from build123d import *

# Parameters (mm, degrees)
SKETCH1_W                    = 370
SKETCH1_H                    = 180
BOSS_EXTRUDE1_DEPTH          = 18
CONVERT_SOLID1_START         = -90
CONVERT_SOLID1_DEPTH         = 180
CONVERT_SOLID1_START_2       = -92
CONVERT_SOLID1_2_DEPTH       = 3.5
CONVERT_SOLID1_START_3       = 88.5
CONVERT_SOLID1_3_DEPTH       = 3.5
CONVERT_SOLID1_START_4       = -88.5
CONVERT_SOLID1_4_DEPTH       = 177
CONVERT_SOLID1_START_5       = -89
CONVERT_SOLID1_5_OUTLINE_W   = 367
CONVERT_SOLID1_5_OUTLINE_H   = 2
CONVERT_SOLID1_5_OUTLINE_W_2 = 2
CONVERT_SOLID1_5_OUTLINE_H_2 = 34.5
CONVERT_SOLID1_5_DEPTH       = 178
CONVERT_SOLID1_START_6       = -89.292893219
CONVERT_SOLID1_6_OUTLINE_W   = 2
CONVERT_SOLID1_6_OUTLINE_H   = 34.5
CONVERT_SOLID1_6_DEPTH       = 178.585786438
CONVERT_SOLID1_START_7       = -183.5
CONVERT_SOLID1_7_DEPTH       = 367
CONVERT_SOLID1_START_8       = -184.292893219
CONVERT_SOLID1_8_OUTLINE_W   = 2
CONVERT_SOLID1_8_OUTLINE_H   = 34.5
CONVERT_SOLID1_8_DEPTH       = 368.585786438
SKETCH6_W                    = 160
SKETCH6_H                    = 140
CUT_EXTRUDE1_DEPTH           = 36


with BuildPart() as part:
    # Sketch1 → Boss-Extrude1 (new, symmetric)
    with BuildSketch(Plane.XY):
        Rectangle(SKETCH1_W, SKETCH1_H)
    extrude(amount=BOSS_EXTRUDE1_DEPTH, both=True)

    # Convert-Solid1: read off the stored shape, not the designer's step
    # Convert-Solid1 outline → Convert-Solid1 (cut)
    with BuildSketch(Plane(origin=(0, 0, 0), x_dir=(1, 0, 0), z_dir=(0, 1, 0)).offset(CONVERT_SOLID1_START)):
        with BuildLine():
            ThreePointArc((-184, 18), (-184.707106781, 17.707106781), (-185, 17))
            Line((-185, 17), (-185, -18))
            Line((-185, -18), (185, -18))
            Line((185, -18), (185, 17))
            ThreePointArc((185, 17), (184.707106781, 17.707106781), (184, 18))
            Line((184, 18), (-184, 18))
        make_face()
    extrude(amount=CONVERT_SOLID1_DEPTH, mode=Mode.SUBTRACT)

    # Convert-Solid1 2 outline → Convert-Solid1 2 (cut)
    with BuildSketch(Plane(origin=(0, 0, 0), x_dir=(1, 0, 0), z_dir=(0, 1, 0)).offset(CONVERT_SOLID1_START_2)):
        with BuildLine():
            ThreePointArc((-185, 17), (-184.707106781, 17.707106781), (-184, 18))
            Line((-184, 18), (-185, 18))
            Line((-185, 18), (-185, 17))
        make_face()
        with BuildLine():
            Line((185, 18), (184, 18))
            ThreePointArc((184, 18), (184.707106781, 17.707106781), (185, 17))
            Line((185, 17), (185, 18))
        make_face()
    extrude(amount=CONVERT_SOLID1_2_DEPTH, mode=Mode.SUBTRACT)

    # Convert-Solid1 3 outline → Convert-Solid1 3 (cut)
    with BuildSketch(Plane(origin=(0, 0, 0), x_dir=(1, 0, 0), z_dir=(0, 1, 0)).offset(CONVERT_SOLID1_START_3)):
        with BuildLine():
            ThreePointArc((-185, 17), (-184.707106781, 17.707106781), (-184, 18))
            Line((-184, 18), (-185, 18))
            Line((-185, 18), (-185, 17))
        make_face()
        with BuildLine():
            Line((185, 18), (184, 18))
            ThreePointArc((184, 18), (184.707106781, 17.707106781), (185, 17))
            Line((185, 17), (185, 18))
        make_face()
    extrude(amount=CONVERT_SOLID1_3_DEPTH, mode=Mode.SUBTRACT)

    # Convert-Solid1 4 outline → Convert-Solid1 4 (add)
    with BuildSketch(Plane(origin=(0, 0, 0), x_dir=(1, 0, 0), z_dir=(0, 1, 0)).offset(CONVERT_SOLID1_START_4)):
        with BuildLine():
            Line((185, 18), (185, -18))
            Line((185, -18), (187, -18))
            Line((187, -18), (187, 17))
            ThreePointArc((187, 17), (186.121320344, 19.121320344), (184, 20))
            Line((184, 20), (-184, 20))
            ThreePointArc((-184, 20), (-186.121320344, 19.121320344), (-187, 17))
            Line((-187, 17), (-187, -18))
            Line((-187, -18), (-185, -18))
            Line((-185, -18), (-185, 18))
            Line((-185, 18), (185, 18))
        make_face()
    extrude(amount=CONVERT_SOLID1_4_DEPTH)

    # Convert-Solid1 5 outline → Convert-Solid1 5 (add)
    with BuildSketch(Plane(origin=(0, 0, 0), x_dir=(1, 0, 0), z_dir=(0, 1, 0)).offset(CONVERT_SOLID1_START_5)):
        with Locations((0, 19)):
            Rectangle(CONVERT_SOLID1_5_OUTLINE_W, CONVERT_SOLID1_5_OUTLINE_H)
        with Locations((-186, -0.75)):
            Rectangle(CONVERT_SOLID1_5_OUTLINE_W_2, CONVERT_SOLID1_5_OUTLINE_H_2)
        with Locations((186, -0.75)):
            Rectangle(CONVERT_SOLID1_5_OUTLINE_W_2, CONVERT_SOLID1_5_OUTLINE_H_2)
    extrude(amount=CONVERT_SOLID1_5_DEPTH)

    # Convert-Solid1 6 outline → Convert-Solid1 6 (add)
    with BuildSketch(Plane(origin=(0, 0, 0), x_dir=(1, 0, 0), z_dir=(0, 1, 0)).offset(CONVERT_SOLID1_START_6)):
        with Locations((-186, -0.75)):
            Rectangle(CONVERT_SOLID1_6_OUTLINE_W, CONVERT_SOLID1_6_OUTLINE_H)
        with Locations((186, -0.75)):
            Rectangle(CONVERT_SOLID1_6_OUTLINE_W, CONVERT_SOLID1_6_OUTLINE_H)
    extrude(amount=CONVERT_SOLID1_6_DEPTH)

    # Convert-Solid1 7 outline → Convert-Solid1 7 (add)
    with BuildSketch(Plane.YZ.offset(CONVERT_SOLID1_START_7)):
        with BuildLine():
            Line((92, -17), (92, 18))
            Line((92, 18), (90, 18))
            Line((90, 18), (90, -17))
            ThreePointArc((90, -17), (89.707106781, -17.707106781), (89, -18))
            Line((89, -18), (89, -20))
            ThreePointArc((89, -20), (91.121320344, -19.121320344), (92, -17))
        make_face()
        with BuildLine():
            Line((-92, 18), (-92, -17))
            ThreePointArc((-92, -17), (-91.121320344, -19.121320344), (-89, -20))
            Line((-89, -20), (-89, -18))
            ThreePointArc((-89, -18), (-89.707106781, -17.707106781), (-90, -17))
            Line((-90, -17), (-90, 18))
            Line((-90, 18), (-92, 18))
        make_face()
    extrude(amount=CONVERT_SOLID1_7_DEPTH)

    # Convert-Solid1 8 outline → Convert-Solid1 8 (add)
    with BuildSketch(Plane.YZ.offset(CONVERT_SOLID1_START_8)):
        with Locations((91, 0.75)):
            Rectangle(CONVERT_SOLID1_8_OUTLINE_W, CONVERT_SOLID1_8_OUTLINE_H)
        with Locations((-91, 0.75)):
            Rectangle(CONVERT_SOLID1_8_OUTLINE_W, CONVERT_SOLID1_8_OUTLINE_H)
    extrude(amount=CONVERT_SOLID1_8_DEPTH)

    # Sketch6 → Cut-Extrude1 (cut)
    with BuildSketch(Plane.XY.offset(-18)):
        Rectangle(SKETCH6_W, SKETCH6_H)
    extrude(amount=-CUT_EXTRUDE1_DEPTH, mode=Mode.SUBTRACT)


solid = part.part
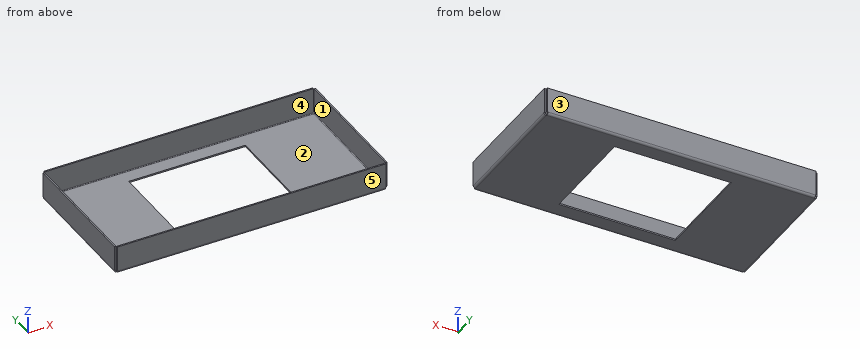
Input: part model. Units: mm. Frame: model coordinates. Face numbers are marked on the shaded views. A direction names the side the tool comes from. Round coordinates to 2 decimals unless told otherwise and drop trailing zeros. Write each loop counter-clockwise with the first axis right and the second up, starting at its lowest first coordinate (ties: lowest second). Pieces come first, ordered by that corner, then holes.
1) Cut plane D-D (x = -138). Return the cut outline in (y, z), then the cut area to 3 significant figures.
2) Ray query, L1, parallel to X at y = 34.5, z = -8.5; L2, parallel to Y at x = -31.5, z = -8; L3, parallel to Z at x = 47, y = 71.5. Return the intervals inside material, ascending.
3) Contact query for flat-ended pins moving along their axis: P1, Ø2, axis at x = -186, z = 0.5, coming from the +Y side; P2, Ø1, axis at y = 24, z = -18.5, coming from the +X side; P3, Ø1.6, axis at y = -90.5, z = -8, coming from the -X side. Output: stop coordinate, or through.
4) Cut plane A-A (x = 37.5). Return the cut outline in (y, z).
5) Draft query along Y for the marked faces 1, 2 and 3. Return one class per face: pulls with the +Y half, pulls with the -Y half, needs draft (parallel to the pull), parting line crosses it, or undercut.
6) Reachability of the marked faces 4 and 5 from +Z, -Z, +X, -X, +Y, -Y: full face, straight path, thin tool, end or side. Return the list, or none.
7) Cut plane B-B (z = -4). Return the cut outline in (x, y), then the cut area to 3 significant figures.
8) Cut plane C-C (y = 44.5). Return the cut outline in (x, z).
Geometry says:
1. outline: (-92, -17) arc R3 ccw to (-89, -20) - (89, -20) arc R3 ccw to (92, -17) - (92, 18) - (90, 18) - (90, -17) arc R1 cw to (89, -18) - (-89, -18) arc R1 cw to (-90, -17) - (-90, 18) - (-92, 18) - close
1. area: 509 mm2
2. L1: x = -187 to -185, 185 to 187
2. L2: y = -92 to -90, 90 to 92
2. L3: z = -20 to -18
3. P1: stops at y = 89.29
3. P2: stops at x = 186.83
3. P3: stops at x = -184.29
4. outline: (-92, -17) arc R3 ccw to (-89, -20) - (-70, -20) - (-70, -18) - (-89, -18) arc R1 cw to (-90, -17) - (-90, 18) - (-92, 18) - close; (70, -20) - (89, -20) arc R3 ccw to (92, -17) - (92, 18) - (90, 18) - (90, -17) arc R1 cw to (89, -18) - (70, -18) - close
5. face 1: needs draft
5. face 2: undercut
5. face 3: pulls with the +Y half
6. face 4: +Z, +X, -X
6. face 5: +Z, -Z, +X, -X, -Y
7. outline: (-187, -89.29) - (-185, -89.29) - (-185, 89.29) - (-187, 89.29) - close; (-184.29, -92) - (184.29, -92) - (184.29, -90) - (-184.29, -90) - close; (-184.29, 90) - (184.29, 90) - (184.29, 92) - (-184.29, 92) - close; (185, -89.29) - (187, -89.29) - (187, 89.29) - (185, 89.29) - close
7. area: 2,190 mm2
8. outline: (-187, -17) arc R3 ccw to (-184, -20) - (-80, -20) - (-80, -18) - (-184, -18) arc R1 cw to (-185, -17) - (-185, 18) - (-187, 18) - close; (80, -20) - (184, -20) arc R3 ccw to (187, -17) - (187, 18) - (185, 18) - (185, -17) arc R1 cw to (184, -18) - (80, -18) - close
